Autodesk Inventor part; units mm, degrees
ref_plane "YZ Plane" through (0, 0, 0) normal (1, 0, 0) x (0, 1, 0)
ref_plane "XZ Plane" through (0, 0, 0) normal (0, 1, 0) x (-1, 0, 0)
ref_plane "XY Plane" through (0, 0, 0) normal (0, 0, 1) x (1, 0, 0)
sketch "Sketch4" plane through (0, 0, 0) normal (0, 0, 1) x (1, 0, 0)
  line L0 (75, -100) -> (-75, -100)
  line L1 (-75, -100) -> (-75, 100)
  line L2 (-75, 100) -> (75, 100)
  line L3 (75, 100) -> (75, -100)
  line L4 (75, -100) -> (-75, 100) construction
  line L5 (-75, -100) -> (75, 100) construction
  line L6 (170, -42) -> (-170, -42)
  line L7 (-170, -42) -> (-170, 42)
  line L8 (-170, 42) -> (170, 42)
  line L9 (170, 42) -> (170, -42)
  line L10 (170, -42) -> (-170, 42) construction
  line L11 (-170, -42) -> (170, 42) construction
  point P0 (0, 0)
  point P1 (0, 0)
  point P2 (0, 0)
  point P3 (75, 42)
  point P4 (-75, 42)
  point P5 (-75, -42)
  point P6 (75, -42)
  dimension "d17" = 84
  dimension "d18" = 340
  dimension "d19" = 150
  dimension "d20" = 200
extrude "Extrusion4" add sketch "Sketch4" along normal mid plane 85
sketch "Sketch5" plane through (0, 0, 0) normal (0, 1, 0) x (-1, 0, 0)
  circle A0 centre (-123, 0) radius 39.5
  circle A1 centre (123, 0) radius 39.5
  line L0 (75, 42.5) -> (-75, 42.5) construction
  line L1 (0, 42.5) -> (0, -42.5) construction
  line L2 (-75, -42.5) -> (75, -42.5) construction
  line L3 (-170, -42.5) -> (-170, 42.5) construction
  line L4 (-170, 0) -> (170, 0) construction
  line L5 (170, -42.5) -> (170, 42.5) construction
  circle A2 centre (-123, 0) radius 31.5
  circle A3 centre (123, 0) radius 31.5
  line L6 (-155, 42.5) -> (-170, 27.5)
  line L7 (-170, -27.5) -> (-155, -42.5)
  line L8 (-170, -42.5) -> (-75, -42.5)
  line L9 (170, 42.5) -> (75, 42.5)
  line L10 (155, 42.5) -> (170, 27.5)
  line L11 (170, -27.5) -> (155, -42.5)
  line L12 (-75, 42.5) -> (-170, 42.5)
  line L13 (75, -42.5) -> (170, -42.5)
  line L14 (-170, 42.5) -> (-170, -42.5)
  line L15 (170, 42.5) -> (170, -42.5)
  point P0 (0, 0)
  point P1 (-170, -27.5)
  dimension "d23" = 79
  dimension "d24" = 246
  dimension "d39" = 63
  dimension "d42" = 15
  dimension "d43" = 45
extrude "Extrusion5" add sketch "Sketch5" against normal blind 32 from surface at -42 contours A0 | A1 | A2 | A3
sketch "Sketch6" plane through (0, 0, 0) normal (0, 0, 1) x (1, 0, 0)
  line L0 (147, 15) -> (-147, 15)
  line L1 (-147, 15) -> (-147, -15)
  line L2 (-147, -15) -> (147, -15)
  line L3 (147, -15) -> (147, 15)
  line L4 (147, 15) -> (-147, -15) construction
  line L5 (-147, 15) -> (147, -15) construction
  line L6 (-60, 85) -> (60, 85)
  line L7 (60, 85) -> (60, -85)
  line L8 (60, -85) -> (-60, -85)
  line L9 (-60, -85) -> (-60, 85)
  line L10 (-60, 85) -> (60, -85) construction
  line L11 (60, 85) -> (-60, -85) construction
  line L12 (75, -100) -> (-75, -100)
  line L13 (-75, 42) -> (-75, 100)
  line L14 (-170, -42) -> (-170, 42)
  line L15 (-75, -42) -> (-170, -42)
  point P0 (0, 0)
  point P1 (-60, -15)
  point P2 (60, -15)
  point P3 (60, 15)
  point P4 (-60, 15)
  dimension "d27" = 15
  dimension "d28" = 15
  dimension "d29" = 23
  dimension "d30" = 27
  dimension "d46" = 30
extrude "Extrusion6" cut sketch "Sketch6" along normal mid plane 55
extrude "Extrusion8" cut sketch "Sketch5" against normal through all both and the other way through all contours L7 L8 L14 | L6 L14 L12 | L15 L10 L9 | L15 L13 L11
mirror "Mirror1" about plane through (0, 0, 0) normal (0, 1, 0) of "Extrusion5"
equation "\"d21\" = body_thickness"
equation "\"d27\" = wall_thickness"
equation "\"d28\" = wall_thickness"
equation "\"d31\" = body_thickness - 2 * wall_thickness"
equation "\"wall_thickness\" = 15"
equation "\"body_thickness\" = 85"
properties part number "body_inventor"
Work out the finished part from the listing and answer in its coordinate system (mm). A direction names the side the tool comes from. Round coordinates to 2 decimals unless told otherwise and drop trailing zeros. Loops run counter-clockwise (first coordinate to the right, second up) from the corner with the lowest first, then second, coordinate; pieces in that order, holes last. Notation, with made-up numbers: (-27.75, 9.25) -> (-18.75, 9.25) arc R32 ccw to (-18.75, 37.25) -> close; hole circle Ø2 at (79, 54.5). An arc over 180 degrees is marked (long way). Write each question's results on one line, items separated by ' | '. Start each with the question number.
1. Section B-B (x = -123) is taken. Determine the outline of the cut face in (y, z).
2. Section A-A (y = 11) is taken. Determine the outline of the cut face in (x, z), plus the area to 3 significant figures.
3. Section D-D (x = -14.5) is taken. Determine the outline of the cut face in (y, z).
4. A tool of negligible diameter and unlimited length cuts with its end or side. For faces 4 (the face through (-111, -42, -38)), 5 (the face through (-60, 50, 0)), 6 (the face through (-124, 74, 1)), 7 (the face through (-112.6, 42, -38.4)), 8 (the face through (-122, -74, 1)), from which of +Z, -Z, +X, -X, +Y, -Y can it reach the whole face along a straight path? Write none if from no direction.
5. Find the intervals of material crossed by probe 1 along X at (y, z) = (66, 3); probe 2 along X at (y, z) = (-9, -22); probe 3 along Y at (x, z) = (36.5, -26.5), in increasing order. Write a range as from..to.
6. For a pull along X with two mould halves and no side action, classify faces 1 (the face through (124, -74, 1)), 2 (the face through (170, 1, 0)), 3 (the face through (-103, 15, 0)) as +X half, -X half, draft (parallel to the pull), parting line (faces both ways), or undercut.
7. Section C-C (y = 36) is taken. Determine the outline of the cut face in (x, z), plus the area to 4 significant figures.
8. Given pin 1 Ø1.5 at (y, z) = (46, 32) entering from +X; pin 2 Ø1.5 at (x, z) = (98.5, 26) entering from -Y; pin 3 Ø23.5 at (x, z) = (-110, -9) entering from +Y, each flat-ended and moving along its own axis, determine where each tip first touches the part or whether it passes through.
Evaluation:
1) outline: (-74, -39.5) -> (-42, -39.5) -> (-42, -42.5) -> (42, -42.5) -> (42, -39.5) -> (74, -39.5) -> (74, 39.5) -> (42, 39.5) -> (42, 42.5) -> (-42, 42.5) -> (-42, 39.5) -> (-74, 39.5) -> close; hole (-15, -27.5) -> (15, -27.5) -> (15, 27.5) -> (-15, 27.5) -> close
2) outline: (-170, -27.5) -> (-155, -42.5) -> (155, -42.5) -> (170, -27.5) -> (170, 27.5) -> (155, 42.5) -> (-155, 42.5) -> (-170, 27.5) -> close; hole (-147, -27.5) -> (147, -27.5) -> (147, 27.5) -> (-147, 27.5) -> close | area: 12,300 mm2
3) outline: (-100, -42.5) -> (100, -42.5) -> (100, 42.5) -> (-100, 42.5) -> close; hole (-85, -27.5) -> (85, -27.5) -> (85, 27.5) -> (-85, 27.5) -> close
4) face 4: -Y | face 5: none | face 6: +Z, -Z, -X, +Y | face 7: +Y | face 8: +Z, -Z, -X, -Y
5) probe 1: x = -162.39..-83.61, -75..-60, 60..75, 83.61..162.39 | probe 2: x = -170..-147, 147..170 | probe 3: y = -100..-85, 85..100
6) face 1: draft | face 2: +X half | face 3: undercut
7) outline: (-170, -27.5) -> (-155, -42.5) -> (155, -42.5) -> (170, -27.5) -> (170, 27.5) -> (155, 42.5) -> (-155, 42.5) -> (-170, 27.5) -> close; hole (-60, -27.5) -> (60, -27.5) -> (60, 27.5) -> (-60, 27.5) -> close | area: 21,850 mm2
8) pin 1: stops at x = 147.16 | pin 2: stops at y = -74 | pin 3: stops at y = 74
